Drawing for the job (mm, zero at the part's lowest x, y, z). Round coordinates to 2 decimals unless told otherwise and drop trailing zeros. Loops run counter-clockwise (first coordinate to the right, second up) from the corner with the lowest first, then second, coordinate; pieces in that order, holes last. Notation, with made-up numbers: (58.5, -11) -> (62.5, -11) arc R17 cw to (62.5, 6) -> close; hole circle Ø8 at (-6, -2.5). An arc over 180 degrees is marked (long way). Put each result on its own line as item: value. Start each with the question number.
Item 1: Cut at A-A, the plane y = 22. List the corners of the cut face in (x, z), plus the area to 3 significant figures.
Item 2: Drill centre lines: probe 1 along Y at (x, z) = (22, 0.5); probe 2 along Y at (x, z) = (22, 1.25); probe 3 along X at (y, z) = (10, 1.3). Where is each one in solid material? Low to high. Write a range as [from, to].
Item 3: Flat gauge pins, fed straight in: pin 1 Ø1 at (y, z) = (37.5, 0.5) entering from -X; pin 2 Ø1 at (x, z) = (16.5, 1.5) entering from +Y. Where does each tip first touch, or does it go through?
Item 4: Pull direction Y, two halves, no side cores. Call the marked faces 1 and 2: +Y half, -Y half, draft (parallel to the pull), parting line (faces both ways), or undercut.
Item 5: Cut at C-C, the plane z = 0.45. List the corners of the cut face in (x, y).
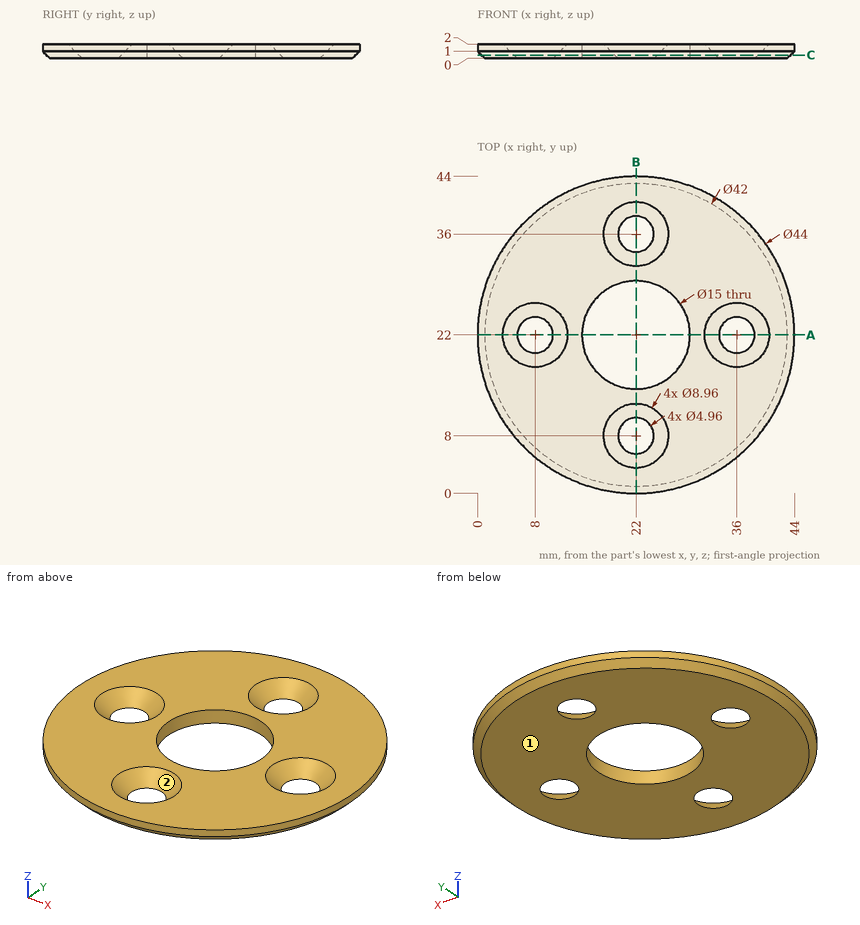
Reply:
1. outline: (0, 1) -> (1, 0) -> (5.52, 0) -> (3.52, 2) -> (0, 2) -> close; (10.48, 0) -> (14.5, 0) -> (14.5, 2) -> (12.48, 2) -> close; (29.5, 0) -> (33.52, 0) -> (31.52, 2) -> (29.5, 2) -> close; (38.48, 0) -> (43, 0) -> (44, 1) -> (44, 2) -> (40.48, 2) -> close
1. area: 29.2 mm^2
2. probe 1: y = [0.5, 5.02], [10.98, 14.5], [29.5, 33.02], [38.98, 43.5]
2. probe 2: y = [0, 4.27], [11.73, 14.5], [29.5, 32.27], [39.73, 44]
2. probe 3: x = [3.56, 18.79], [25.21, 40.44]
3. pin 1: stops at x = 6.23
3. pin 2: stops at y = 43.42
4. face 1: draft
4. face 2: undercut
5. outline: circle Ø42.9 at (22, 22); hole circle Ø5.86 at (8, 22); hole circle Ø15 at (22, 22); hole circle Ø5.86 at (22, 8); hole circle Ø5.86 at (22, 36); hole circle Ø5.86 at (36, 22)
